from build123d import *

# Parameters (mm, degrees)
EXTRUDE_1_DEPTH      = 5
HOLE_WIZARD_M3_D     = 2.5
HOLE_WIZARD_M3_DEPTH = 7.5
HOLE_WIZARD_M3_TIP   = 0.751075774


with BuildPart() as part:
    # 草图1 → 凸台-拉伸1 (new, symmetric)
    with BuildSketch(Plane.XY):
        with BuildLine():
            Line((-2.8, 4.7), (2.8, 4.7))
            ThreePointArc((2.8, 4.7), (2.941421356, 4.641421356), (3, 4.5))
            Line((3, 4.5), (3, 3.2))
            Line((3, 3.2), (4.5, 3.2))
            ThreePointArc((4.5, 3.2), (4.641421356, 3.141421356), (4.7, 3))
            Line((4.7, 3), (4.7, 2.45))
            ThreePointArc((4.7, 2.45), (4.047583818, 0.994220712), (2.8, 0))
            Line((2.8, 0), (-2.8, 0))
            ThreePointArc((-2.8, 0), (-4.047583818, 0.994220712), (-4.7, 2.45))
            Line((-4.7, 2.45), (-4.7, 3))
            ThreePointArc((-4.7, 3), (-4.641421356, 3.141421356), (-4.5, 3.2))
            Line((-4.5, 3.2), (-3, 3.2))
            Line((-3, 3.2), (-3, 4.5))
            ThreePointArc((-3, 4.5), (-2.941421356, 4.641421356), (-2.8, 4.7))
        make_face()
    extrude(amount=EXTRUDE_1_DEPTH, both=True)

    # M3螺纹孔
    with Locations(Plane.ZX.offset(4.7)):
        with Locations((0, 0)):
            Hole(HOLE_WIZARD_M3_D / 2, depth=HOLE_WIZARD_M3_DEPTH)
            with Locations((0, 0, -(HOLE_WIZARD_M3_DEPTH + HOLE_WIZARD_M3_TIP / 2))):  # 118° drill point
                Cone(0, HOLE_WIZARD_M3_D / 2, HOLE_WIZARD_M3_TIP, mode=Mode.SUBTRACT)


solid = part.part
The model under review builds one solid part; all positions refer to its coordinate system, in mm. A direction names the side the tool comes from. Round coordinates to 2 decimals unless told otherwise and drop trailing zeros. Loops run counter-clockwise (first coordinate to the right, second up) from the corner with the lowest first, then second, coordinate; pieces in that order, holes last. Notation, with made-up numbers: (46, 65) -> (105, 65) arc R31 cw to (105, 97) -> close; hole circle Ø8 at (-10.5, -12). An arc over 180 degrees is marked (long way). Return JSON: item names as keys, results as strings.
(1) Add section C-C on y = 3.9. Write out the cut boundary in (x, z), plus the area to 3 significant figures.
Solved:
{"outline": "(-3, -5) -> (3, -5) -> (3, 5) -> (-3, 5) -> close; hole circle Ø2.5 at (0, 0)", "area": "55.1 mm2"}
(2) For pin 1 (1.2 mm diameter, centred on x = 4, z = -2, fed in from +Y), flat-tipped, find the tip position at first contact; note if it passes through.
Solved:
{"pin 1": "y = 3.2"}
(3) Add section B-B on x = 0. Write out the cut boundary in (y, z), plus the area to 4 significant figures.
Solved:
{"outline": "(0, -5) -> (4.7, -5) -> (4.7, -1.25) -> (0, -1.25) -> close; (0, 1.25) -> (4.7, 1.25) -> (4.7, 5) -> (0, 5) -> close", "area": "35.25 mm2"}
(4) The part is to be moulded in two halves that separate along X. For faces 4 (the cylindrical face through (-4.034, 0.976, 0.07)), 5 (the flat face through (1, 0, 1)), 6 (the cylindrical face through (-1.22, 2.32, 0.27)), say which applies: released by +X, released by -X, zero draft, split by the parting line, or undercut.
Solved:
{"face 4": "released by -X", "face 5": "zero draft", "face 6": "undercut"}
(5) For line 1 (X direction, y = 3, z = 0); line 2 (X direction, y = 3.5, z = 0); line 3 (Z direction, x = -0.5, y = 4.05), list the stretches that pass through material, from the lowest coordinate up.
Solved:
{"line 1": "-4.7 to -1.25, 1.25 to 4.7", "line 2": "-3 to -1.25, 1.25 to 3", "line 3": "-5 to -1.15, 1.15 to 5"}
(6) Add section A-A on z = 0. Write out the cut boundary in (x, y).
Solved:
{"outline": "(-4.7, 2.45) arc R3.38 ccw to (-2.8, 0) -> (-1.25, 0) -> (-1.25, 4.7) -> (-2.8, 4.7) arc R0.2 ccw to (-3, 4.5) -> (-3, 3.2) -> (-4.5, 3.2) arc R0.2 ccw to (-4.7, 3) -> close; (1.25, 0) -> (2.8, 0) arc R3.38 ccw to (4.7, 2.45) -> (4.7, 3) arc R0.2 ccw to (4.5, 3.2) -> (3, 3.2) -> (3, 4.5) arc R0.2 ccw to (2.8, 4.7) -> (1.25, 4.7) -> close"}
(7) For faces 1 (the flat face through (3, 4, 0)), 2 (the flat face through (0, 2, 5)), 3 (the flat face through (-3, 4, 0)), list the 3-axis set-ups (+Z, -Z, +X, -X, +Y, -Y) from which the entire face can be reached by the end or side of a thin tool; tool diameter is ignored.
Solved:
{"face 1": "+Z, -Z, +X, +Y", "face 2": "+Z, +X, -X, +Y, -Y", "face 3": "+Z, -Z, -X, +Y"}
(8) Add section D-D on z = 1. Write out the cut boundary in (x, y), plus the area to 3 significant figures.
Solved:
{"outline": "(-4.7, 2.45) arc R3.38 ccw to (-2.8, 0) -> (-0.75, 0) -> (-0.75, 4.7) -> (-2.8, 4.7) arc R0.2 ccw to (-3, 4.5) -> (-3, 3.2) -> (-4.5, 3.2) arc R0.2 ccw to (-4.7, 3) -> close; (0.75, 0) -> (2.8, 0) arc R3.38 ccw to (4.7, 2.45) -> (4.7, 3) arc R0.2 ccw to (4.5, 3.2) -> (3, 3.2) -> (3, 4.5) arc R0.2 ccw to (2.8, 4.7) -> (0.75, 4.7) -> close", "area": "28.9 mm2"}
